from build123d import *

# Parameters (mm, degrees)
F1_DEPTH = 180
F2_R     = 31.542376
F3_DEPTH = 20


with BuildPart() as f1:
    # F0 (on Front) → F1 (new body)
    with BuildSketch(Plane.XZ):
        Polygon((7.28047, 6.002584), (7.28047, 29.945172), (-7.141014, 7.986175), (-30.399669, -0.422769), (-9.899175, -5.597863), (-1.747458, -28.145044), (4.973325, -9.345488), (29.653051, -0.422769), align=None)
    extrude(amount=F1_DEPTH)

    # F2 (on face) → F3 (join)
    with BuildSketch(Plane.XZ):
        Circle(F2_R)
    extrude(amount=F3_DEPTH)


solid = f1.part
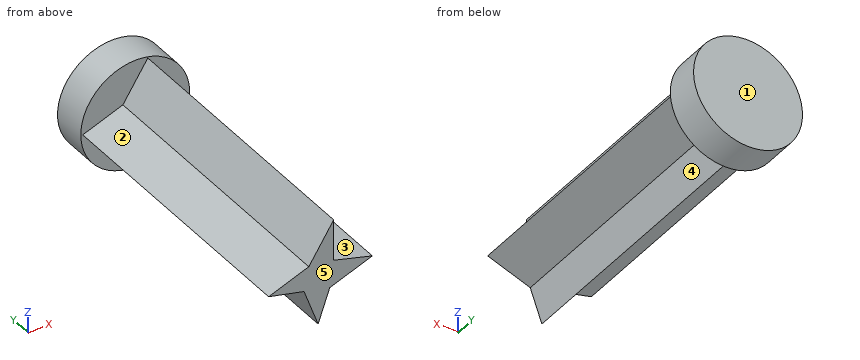
Model file for the job. Use its own axes, mm. Face numbers are marked on the shaded views. A direction names the side the tool comes from. Round coordinates to 2 decimals unless told otherwise and drop trailing zeros. Order: outer loops, then holes, each group sorted by start corner. A loop starts at its lowest first (then second) coordinate and runs counter-clockwise, first axis right, second up.
(1) Band-saw the part on B-B (z = 21.5). List the corners of the cut face in (x, y), then the cut area to 3 significant figures.
(2) 3-axis set-ups, long thin cutter, end or side, ignore diameter. For the marked faces 1, 2, 3, 4 and 5: which of +Z, -Z, +X, -X, +Y, -Y reach the whole face in a straight line?
(3) Pin check, flat tips, straight feed: pin 1 (4 mm diameter, centred on x = -2, y = -89, fed in from +Z); pin 2 (2 mm diameter, centred on x = 20, y = -116, fed in from -Z); pin 3 (12 mm diameter, centred on x = 13.5, z = -18.5, fed in from -Y). Stop position of each tip, or through.
(4) Drill centre lines: line 1 (Y direction, x = 6.5, z = -25); line 2 (Z direction, x = 14, y = -63); line 3 (Z direction, x = 27.5, y = -60.5). Where is each one in solid material? Low to high.
(5) Band-saw the part on A-A (y = -57). List the corners of the cut face in (x, z).
Verdict:
1. outline: (-23.08, -20) - (1.73, -20) - (1.73, -180) - (7.28, -180) - (7.28, -20) - (23.08, -20) - (23.08, 0) - (-23.08, 0) - close
1. area: 1,810 mm2
2. face 1: +Z, -Z, +X, -X, +Y
2. face 2: +Z, -X, -Y
2. face 3: +Z, +X, -Y
2. face 4: -Z, +X, -Y
2. face 5: +Z, -Z, +X, -X, -Y
3. pin 1: stops at z = 18.86
3. pin 2: stops at z = -4.27
3. pin 3: stops at y = -20
4. line 1: y = -20 to 0
4. line 2: z = -6.08 to 4.07
4. line 3: z = -1.2 to 0.2
5. outline: (-30.4, -0.42) - (-9.9, -5.6) - (-1.75, -28.15) - (4.97, -9.35) - (29.65, -0.42) - (7.28, 6) - (7.28, 29.95) - (-7.14, 7.99) - close
